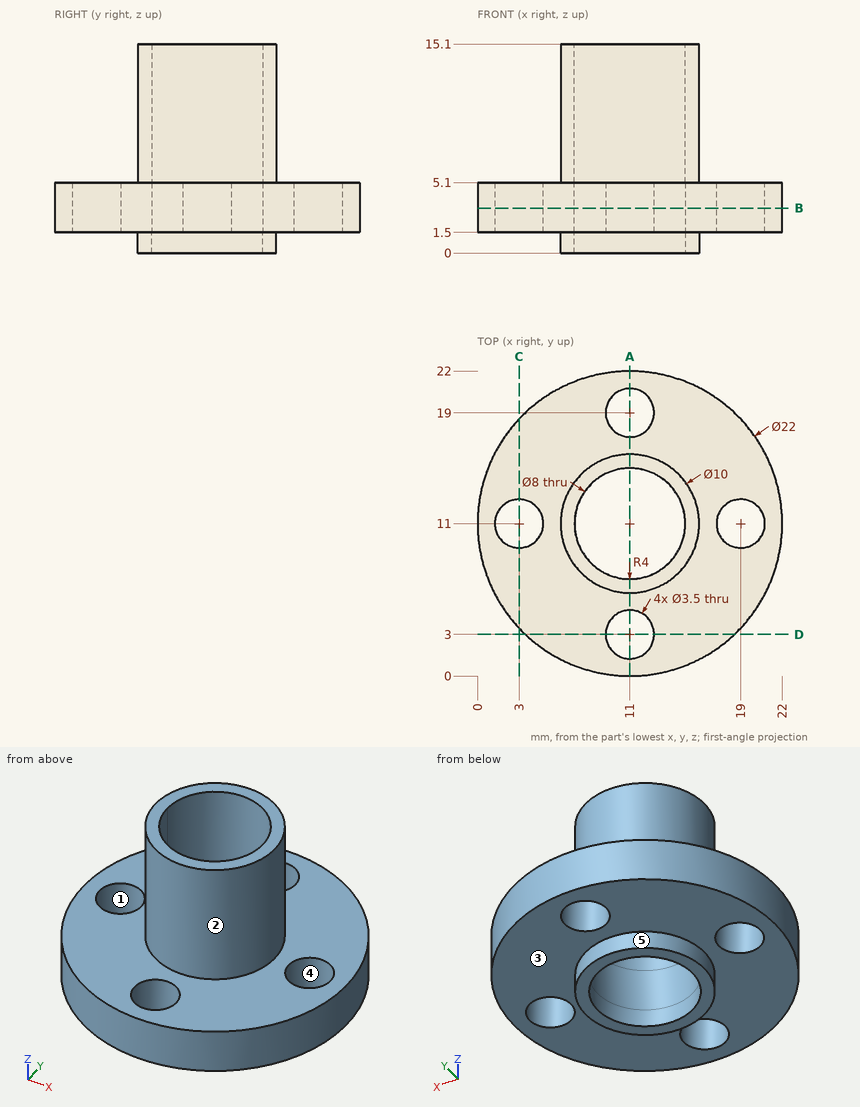
Could you check a few things on this drawing? It's one solid part, dimensions in mm from its lowest x, y, z. A direction names the side the tool comes from. Coordinates: 2 decimals unless noted, no trailing zeros. Order: outer loops, then holes, each group sorted by start corner. A loop starts at its lowest first (then second) coordinate and runs counter-clockwise, first axis right, second up. Notation, with made-up numbers: M -25.75,-40 L 31.25,-40 A20 ccw 31.25,-19 Z; hole C 71.5,70.5 d8. An arc over 180 degrees is marked long. Answer as CSV lines item,"result".
(1) Please list where these lines run through material, in increasing order: L1, parallel to Y at x = 11, z = 2.6; L2, parallel to Z at x = 5.5, y = 5.25; L3, parallel to Y at x = 3, z = 2.65.
Geometry check:
L1,"0 to 1.25, 4.75 to 7, 15 to 17.25, 20.75 to 22"
L2,"1.5 to 5.1"
L3,"3.45 to 9.25, 12.75 to 18.55"
(2) Suppose I cut it at B-B on z = 3.25. Please give me the cut outline in (x, y), plus the area to 3 significant figures.
Geometry check:
outline,"C 11,11 d22; hole C 3,11 d3.5; hole C 11,11 d8; hole C 11,3 d3.5; hole C 11,19 d3.5; hole C 19,11 d3.5"
area,"291 mm^2"
(3) Suppose I cut it at A-A on x = 11. Please give me the cut outline in (y, z).
Geometry check:
outline,"M 0,1.5 L 1.25,1.5 L 1.25,5.1 L 0,5.1 Z; M 4.75,1.5 L 6,1.5 L 6,0 L 7,0 L 7,15.1 L 6,15.1 L 6,5.1 L 4.75,5.1 Z; M 15,0 L 16,0 L 16,1.5 L 17.25,1.5 L 17.25,5.1 L 16,5.1 L 16,15.1 L 15,15.1 Z; M 20.75,1.5 L 22,1.5 L 22,5.1 L 20.75,5.1 Z"
(4) On a 3-axis mill with a long thin cutter (end or side, diameter ignored), from which of +Z, -Z, +X, -X, +Y, -Y can I reach the whole of each face in a straight line? I mean the marked faces 1 and 2. Say none if no direction works.
Geometry check:
face 1,"+Z, -Z"
face 2,"+Z"
(5) Suppose I cut it at C-C on x = 3. Please give me the cut outline in (y, z), plus the area to 3 significant figures.
Geometry check:
outline,"M 3.45,1.5 L 9.25,1.5 L 9.25,5.1 L 3.45,5.1 Z; M 12.75,1.5 L 18.55,1.5 L 18.55,5.1 L 12.75,5.1 Z"
area,"41.8 mm^2"
(6) I'm going to push flat-ended pins straight in: pin 1 (7 mm diameter, centred on x = 11, y = 11, fed in from -Z); pin 2 (8 mm diameter, centred on y = 6.5, z = 11, fed in from -X); pin 3 (5.5 mm diameter, centred on x = 11, y = 19, fed in from -Z); pin 4 (3 mm diameter, centred on x = 11.5, z = 13.5, fed in from -Y). Where does each tip first touch, or does it pass through?
Geometry check:
pin 1,"through"
pin 2,"x = 6.03"
pin 3,"z = 1.5"
pin 4,"y = 6"
(7) If we mould it in two halves opening along Y, with no side actions, what happens to the marked faces 3, 4 and 5? For each: released by +Y, released by -Y, zero draft, split by the parting line, or undercut.
Geometry check:
face 3,"zero draft"
face 4,"undercut"
face 5,"split by the parting line"
